Part print with two shaded views. Sizes in mm from the minimum x, y, z corner. Round coordinates to 2 decimals unless told otherwise and drop trailing zeros. Write each loop counter-clockwise with the first axis right and the second up, starting at its lowest first coordinate (ties: lowest second). Pieces come first, ordered by that corner, then holes. Notation, with made-up numbers: (-16, -19) -> (9, -19) arc R15 ccw to (9, -12) -> close; hole circle Ø4 at (16.25, 44.25). An arc over 180 degrees is marked (long way). Return JSON: item names as keys, results as strings. Group by question number.
(1) Saw through at C-C (z = 32.5). List the corners of the cut face in (x, y).
(2) Saw through at B-B (y = 1.65). List the corners of the cut face in (x, z), plus the area to 3 significant figures.
(3) Drill centre lines: L1, parallel to X at y = 1.9, z = 32.5; L2, parallel to X at y = 1.6, z = 62; L3, parallel to X at y = 2.25, z = 6. Where is each one in solid material? Low to high. Write a range as from..to.
(4) Saw through at D-D (x = 6). List the corners of the cut face in (y, z).
(5) Saw through at A-A (x = 32.5). List the corners of the cut face in (y, z), plus the area to 3 significant figures.
(6) Drop flat-ended pins along their axis: pin 1 Ø1 at (x, y) = (17.5, 2.5) entering from +Z; pin 2 Ø1.5 at (x, y) = (60, 2) entering from +Z; pin 3 Ø1.5 at (y, z) = (1.5, 27.5) entering from -X. Give the stop position or say it passes through.
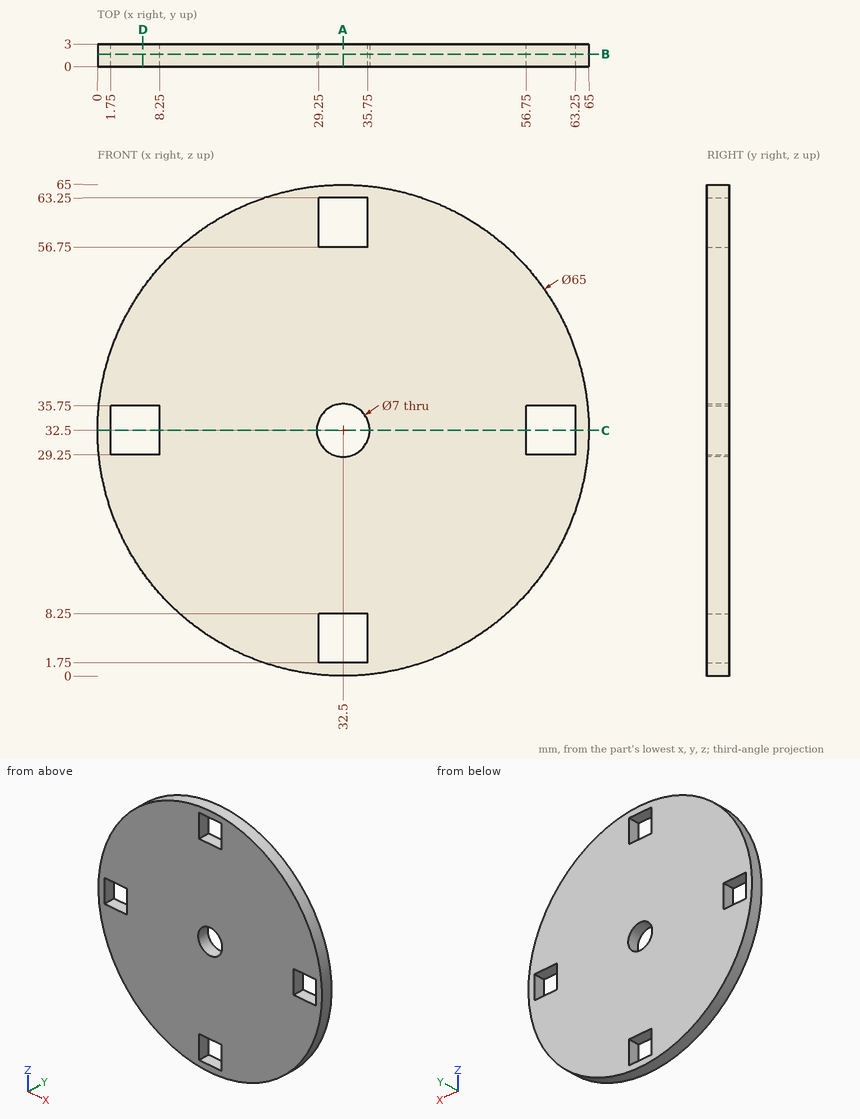
Computed values:
{
 "1": {"outline": "(0, 0) -> (1.75, 0) -> (1.75, 3) -> (0, 3) -> close; (8.25, 0) -> (29, 0) -> (29, 3) -> (8.25, 3) -> close; (36, 0) -> (56.75, 0) -> (56.75, 3) -> (36, 3) -> close; (63.25, 0) -> (65, 0) -> (65, 3) -> (63.25, 3) -> close"},
 "2": {"outline": "circle Ø65 at (32.5, 32.5); hole (1.75, 29.25) -> (8.25, 29.25) -> (8.25, 35.75) -> (1.75, 35.75) -> close; hole circle Ø7 at (32.5, 32.5); hole (29.25, 1.75) -> (35.75, 1.75) -> (35.75, 8.25) -> (29.25, 8.25) -> close; hole (29.25, 56.75) -> (35.75, 56.75) -> (35.75, 63.25) -> (29.25, 63.25) -> close; hole (56.75, 29.25) -> (63.25, 29.25) -> (63.25, 35.75) -> (56.75, 35.75) -> close", "area": "3,110 mm2"},
 "3": {"L1": "0..1.75, 8.25..29, 36..56.75, 63.25..65", "L2": "18.86..29.25, 35.75..46.14", "L3": "13.69..29.25, 35.75..51.31"},
 "4": {"outline": "(0, 13.69) -> (3, 13.69) -> (3, 29.25) -> (0, 29.25) -> close; (0, 35.75) -> (3, 35.75) -> (3, 51.31) -> (0, 51.31) -> close"},
 "5": {"outline": "(0, 0) -> (3, 0) -> (3, 1.75) -> (0, 1.75) -> close; (0, 8.25) -> (3, 8.25) -> (3, 29) -> (0, 29) -> close; (0, 36) -> (3, 36) -> (3, 56.75) -> (0, 56.75) -> close; (0, 63.25) -> (3, 63.25) -> (3, 65) -> (0, 65) -> close", "area": "135 mm2"},
 "6": {"pin 1": "z = 61.59", "pin 2": "z = 50.96", "pin 3": "x = 0.28"}
}
